Here's how the part is built. I have some questions about the finished solid (model axes, mm). A direction names the side the tool comes from. Give positions to 0.01 mm unless a question says otherwise; leave off trailing zeros. Order: outer loops, then holes, each group sorted by start corner. A loop starts at its lowest first (then second) coordinate and runs counter-clockwise, first axis right, second up.
from build123d import *

# Parameters (mm, degrees)
EXTRUDE_1_DEPTH     = 17
SKETCH_2_R          = 2.75
CUT_EXTRUDE_1_DEPTH = 17
SKETCH_3_R          = 2.75
CUT_EXTRUDE_2_DEPTH = 17


with BuildPart() as part:
    # 草图1 → 凸台-拉伸1 (new body)
    with BuildSketch(Plane(origin=(0, 0, 0), x_dir=(1, 0, 0), z_dir=(0, 1, 0))):
        Polygon((80, 0), (0, 0), (56.568542495, 56.568542495), (59.39696962, 53.74011537), (9.656854249, 4), (80, 4), align=None)
    extrude(amount=EXTRUDE_1_DEPTH)

    # 草图2 → 切除-拉伸1 (cut)
    with BuildSketch(Plane(origin=(2.828427125, 0, 2.828427125), x_dir=(0.7071067811865476, 0, -0.7071067811865476), z_dir=(0.7071067811865476, 0, 0.7071067811865476))):
        with Locations((70, 8.5)):
            Circle(SKETCH_2_R)
    extrude(amount=-CUT_EXTRUDE_1_DEPTH, mode=Mode.SUBTRACT)

    # 草图3 → 切除-拉伸2 (cut)
    with BuildSketch(Plane.XY):
        with Locations((70, 8.5)):
            Circle(SKETCH_3_R)
    extrude(amount=-CUT_EXTRUDE_2_DEPTH, mode=Mode.SUBTRACT)


solid = part.part
Q1. If we section it at D-D on x = 22.5: List the corners of the cut face in (y, z) for me, plus the area to 3 significant figures.
Filled sheet:
outline: (0, -22.5) - (17, -22.5) - (17, -16.84) - (0, -16.84) - close; (0, -4) - (17, -4) - (17, 0) - (0, 0) - close
area: 164 mm2
Q2. If we section it at A-A on x = 70: List the corners of the cut face in (y, z) for me.
Filled sheet:
outline: (0, -4) - (5.75, -4) - (5.75, 0) - (0, 0) - close; (11.25, -4) - (17, -4) - (17, 0) - (11.25, 0) - close
Q3. I'm going to push flat-ended pins straight in: P1, Ø1, axis at x = 63, y = 3.5, coming from the +Z side; P2, Ø2, axis at y = 13.5, z = -30.5, coming from the -X side; P3, Ø6, axis at y = 8.5, z = -16.5, coming from the -X side; P4, Ø2, axis at x = 59, y = 11.5, coming from the -Z side. Where does each tip first touch, or does it pass through?
Filled sheet:
P1: stops at z = 0
P2: stops at x = 29.5
P3: stops at x = 13.5
P4: stops at z = -55.14
Q4. If we section it at B-B on y = 3: List the corners of the cut face in (x, z) for me.
Filled sheet:
outline: (0, 0) - (56.57, -56.57) - (59.4, -53.74) - (9.66, -4) - (80, -4) - (80, 0) - close
Q5. I need wall thicknesses on L1, parallel to Y at x = 70, z = -2.6; L2, parallel to Z at x = 28, y = 3.5; L3, parallel to Z at x = 41, y = 11.5. Which ranges of each line are inside material? Lowest first, please.
Filled sheet:
L1: y = 0 to 5.75, 11.25 to 17
L2: z = -28 to -22.34, -4 to 0
L3: z = -41 to -35.34, -4 to 0
Q6. If we section it at C-C on y = 8.5: List the corners of the cut face in (x, z) for me, plus the area to 3 significant figures.
Filled sheet:
outline: (0, 0) - (47.55, -47.55) - (50.38, -44.72) - (9.66, -4) - (67.25, -4) - (67.25, 0) - close; (51.44, -51.44) - (56.57, -56.57) - (59.4, -53.74) - (54.27, -48.61) - close; (72.75, -4) - (80, -4) - (80, 0) - (72.75, 0) - close
area: 557 mm2
Q7. Thinking about a two-plate mould opening in Z: for faces 3 (the face through (37, 17, -3)), 4 (the face through (44, 8, -4)), 5 (the face through (28, 8, -28)), 6 (the face through (52.786, 9.326, -49.918)), which applies, released by +Z, released by -Z, zero draft, split by the parting line, or undercut?
Filled sheet:
face 3: zero draft
face 4: undercut
face 5: released by -Z
face 6: undercut
Q8. For faces 1 (the face through (80, 8, -2)), 2 (the face through (34.875, 8.381, -29.218)), which set-ups out of +Z, -Z, +X, -X, +Y, -Y let a thin tool reach every point of the face, with its end or its side?
Filled sheet:
face 1: +Z, -Z, +X, +Y, -Y
face 2: +X, +Y, -Y
